from build123d import *
from build123d.topology import SkipClean

# Parameters (mm, degrees)
EXTRUDE_1_DEPTH                            = 3.9
EXTRUDE_3_DEPTH                            = 20
EXTRUDE_5_DEPTH                            = 20
FILLET_1_R                                 = 0.25
FILLET_1_OF_MIRROR_2_R                     = 0.25
SKETCH_7_R                                 = 5.5
CUT_EXTRUDE_3_DEPTH                        = 69.146236458
MIRROR_3_AT_THE_SECOND_PLANE_COPY_1_SKET_R = 5.5
MIRROR_3_AT_THE_SECOND_PLANE_COPY_1_DEPTH  = 69.146236458
ESQUISSE1_W                                = 44.6
ESQUISSE1_H                                = 40
ENL_V_MAT_EXTRU_1_DEPTH                    = 1.54
ENL_V_START                                = -27.2
ENL_V_MAT_EXTRU_2_DEPTH                    = 54.4
ENL_V_MAT_EXTRU_2_2_DEPTH                  = 7.2
ENL_V_START_2                              = 20
ENL_V_MAT_EXTRU_2_3_DEPTH                  = 7.2
ESQUISSE3_W                                = 50
ESQUISSE3_H                                = 1.36
ENL_V_MAT_EXTRU_3_DEPTH                    = 64.372466761
ESQUISSE4_W                                = 27.815449133
ESQUISSE4_H                                = 40
ENL_V_MAT_EXTRU_4_DEPTH                    = 54.066651895
ESQUISSE5_R                                = 1.75
ENL_V_MAT_EXTRU_5_DEPTH                    = 54.198396436


# Read off the part's stored shape, not the designer's step: Enl_v. mat.-Extru.2
with BuildPart() as part:
    # Sketch 1 → Extrude 1 (new body)
    with BuildSketch(Plane(origin=(0, 0, 0), x_dir=(1, 0, 0), z_dir=(0, 1, 0))):
        with BuildLine():
            Line((-40.6, -27.2), (40.6, -27.2))
            ThreePointArc((40.6, -27.2), (43.428427125, -26.028427125), (44.6, -23.2))
            Line((44.6, -23.2), (44.6, 23.2))
            ThreePointArc((44.6, 23.2), (43.428427125, 26.028427125), (40.6, 27.2))
            Line((40.6, 27.2), (-40.6, 27.2))
            ThreePointArc((-40.6, 27.2), (-43.428427125, 26.028427125), (-44.6, 23.2))
            Line((-44.6, 23.2), (-44.6, -23.2))
            ThreePointArc((-44.6, -23.2), (-43.428427125, -26.028427125), (-40.6, -27.2))
        make_face()
    extrude(amount=EXTRUDE_1_DEPTH)



with BuildPart() as body_2:
    # Sketch 3 → Extrude 3 (new, symmetric)
    with BuildSketch(Plane.XY):
        with BuildLine():
            Line((-47.815262386, -6.499919999), (-45.841869662, -6.499919999))
            ThreePointArc((-45.841869662, -6.499919999), (-44.821869662, -1.3), (-43.801869662, -6.499919999))
            Line((-43.801869662, -6.499919999), (-41.828476938, -6.499919999))
            ThreePointArc((-41.828476938, -6.499919999), (-44.821869662, -0.1), (-47.815262386, -6.499919999))
        make_face()
    extrude_3 = extrude(amount=EXTRUDE_3_DEPTH, both=True)


with BuildPart() as part_1:
    with SkipClean():  # the faces are left unmerged after this step: merging them gives an invalid solid
        add(part.part)

        add(body_2.part)  # Extrude 5 merges body 2
        # Sketch 5 → Extrude 5 (add, symmetric)
        with BuildSketch(Plane.XY):
            with BuildLine():
                Line((-36.641600827, 0.870983001), (-34.6, 0))
                ThreePointArc((-34.6, 0), (-38.684888017, -1.351535806), (-41.039960555, -4.952451312))
                Line((-41.039960555, -4.952451312), (-42.295442046, -4.952451312))
                ThreePointArc((-42.295442046, -4.952451312), (-44.821869662, -1.3), (-47.348297278, -4.952451312))
                Line((-47.348297278, -4.952451312), (-48.60377877, -4.952451312))
                ThreePointArc((-48.60377877, -4.952451312), (-44.732839073, 2.293818231), (-36.641600827, 0.870983001))
            make_face()
        extrude_5 = extrude(amount=EXTRUDE_5_DEPTH, both=True)

    # Fillet 1
    fillet_1_edges = [part_1.edges().sort_by_distance(p)[0] for p in [
        (-45.841869662, -6.499919999, 0),
        (-43.801869662, -6.499919999, 0),
    ]]
    fillet(fillet_1_edges, radius=FILLET_1_R)

    # Mirror 1: Extrude 5 across plane
    with SkipClean():  # the faces are left unmerged after this step: merging them gives an invalid solid
        add(extrude_5.mirror(Plane(origin=(0, 0, 0), x_dir=(0, 0, 1), z_dir=(1, 0, 0))))

    # Mirror 2: Extrude 3 across plane
    with SkipClean():  # the faces are left unmerged after this step: merging them gives an invalid solid
        add(extrude_3.mirror(Plane(origin=(0, 0, 0), x_dir=(0, 0, 1), z_dir=(1, 0, 0))))

    # Fillet 1 of Mirror 2
    fillet_1_of_mirror_2_edges = [part_1.edges().sort_by_distance(p)[0] for p in [
        (45.841869662, -6.499919999, 0),
        (43.801869662, -6.499919999, 0),
    ]]
    fillet(fillet_1_of_mirror_2_edges, radius=FILLET_1_OF_MIRROR_2_R)

    # Sketch 7 → Cut-Extrude 3 (cut, through all)
    with SkipClean():  # the faces are left unmerged after this step: merging them gives an invalid solid
        with BuildSketch(Plane.XY.offset(20)):
            with Locations((-45, -4)):
                Circle(SKETCH_7_R)
        cut_extrude_3 = extrude(amount=CUT_EXTRUDE_3_DEPTH, mode=Mode.SUBTRACT)

    # Mirror 3: Cut-Extrude 3 across plane
    with SkipClean():  # the faces are left unmerged after this step: merging them gives an invalid solid
        add(cut_extrude_3.mirror(Plane(origin=(0, 0, 0), x_dir=(0, 0, 1), z_dir=(1, 0, 0))), mode=Mode.SUBTRACT)

    # Mirror 3 at the second plane: Cut-Extrude 3 across plane
    with SkipClean():  # the faces are left unmerged after this step: merging them gives an invalid solid
        add(cut_extrude_3.mirror(Plane.XY), mode=Mode.SUBTRACT)

    # Mirror 3 at the second plane copy 1 sket → Mirror 3 at the second plane copy 1 (cut, through all)
    with SkipClean():  # the faces are left unmerged after this step: merging them gives an invalid solid
        with BuildSketch(Plane(origin=(0, 0, -20), x_dir=(-1, 0, 0), z_dir=(0, 0, -1))):
            with Locations((-45, -4)):
                Circle(MIRROR_3_AT_THE_SECOND_PLANE_COPY_1_SKET_R)
        extrude(amount=MIRROR_3_AT_THE_SECOND_PLANE_COPY_1_DEPTH, mode=Mode.SUBTRACT)

    # Esquisse1 → Enl_v. mat.-Extru.1 (cut)
    with SkipClean():  # the faces are left unmerged after this step: merging them gives an invalid solid
        with BuildSketch(Plane(origin=(0, 3.9, 0), x_dir=(1, 0, 0), z_dir=(0, 1, 0))):
            with Locations((-22.3, 0)):
                Rectangle(ESQUISSE1_W, ESQUISSE1_H)
        extrude(amount=-ENL_V_MAT_EXTRU_1_DEPTH, mode=Mode.SUBTRACT)

    # Enl_v. mat.-Extru.2 outline → Enl_v. mat.-Extru.2 (cut)
    with SkipClean():  # the faces are left unmerged after this step: merging them gives an invalid solid
        with BuildSketch(Plane.XY.offset(ENL_V_START)):
            with BuildLine():
                Line((0, 3.9), (0, 0))
                Line((0, 0), (34.815449133, 0))
                ThreePointArc((34.815449133, 0), (38.762946625, -1.412512906), (41.03576021, -4.935614887))
                ThreePointArc((41.03576021, -4.935614887), (41.343051607, -5.76290242), (41.828476938, -6.499919999))
                Line((41.828476938, -6.499919999), (42.913896916, -6.499919999))
                ThreePointArc((42.913896916, -6.499919999), (43.148596508, -6.33603679), (43.075589522, -6.059248812))
                ThreePointArc((43.075589522, -6.059248812), (44.821869662, -1.3), (46.568149802, -6.059248812))
                ThreePointArc((46.568149802, -6.059248812), (46.495142816, -6.33603679), (46.729842408, -6.499919999))
                Line((46.729842408, -6.499919999), (47.815262386, -6.499919999))
                ThreePointArc((47.815262386, -6.499919999), (48.623960619, -4.868391822), (48.60377877, -3.047548688))
                ThreePointArc((48.60377877, -3.047548688), (47.293490745, 0.166982283), (44.6, 2.356770326))
                Line((44.6, 2.356770326), (44.6, 3.9))
                Line((44.6, 3.9), (0, 3.9))
            make_face()
        extrude(amount=ENL_V_MAT_EXTRU_2_DEPTH, mode=Mode.SUBTRACT)

    # Enl_v. mat.-Extru.2 2 outline → Enl_v. mat.-Extru.2 2 (cut)
    with SkipClean():  # the faces are left unmerged after this step: merging them gives an invalid solid
        with BuildSketch(Plane.XY.offset(ENL_V_START)):
            with BuildLine():
                Line((0, 0), (0, 3.9))
                Line((0, 3.9), (-44.6, 3.9))
                Line((-44.6, 3.9), (-44.60000095, 1.48543533))
                ThreePointArc((-44.60000095, 1.48543533), (-42.784348631, 1.033973481), (-41.225082782, 0))
                Line((-41.225082782, 0), (0, 0))
            make_face()
        extrude(amount=ENL_V_MAT_EXTRU_2_2_DEPTH, mode=Mode.SUBTRACT)

    # Enl_v. mat.-Extru.2 3 outline → Enl_v. mat.-Extru.2 3 (cut)
    with SkipClean():  # the faces are left unmerged after this step: merging them gives an invalid solid
        with BuildSketch(Plane.XY.offset(ENL_V_START_2)):
            with BuildLine():
                Line((0, 0), (0, 3.9))
                Line((0, 3.9), (-44.6, 3.9))
                Line((-44.6, 3.9), (-44.60000095, 1.48543533))
                ThreePointArc((-44.60000095, 1.48543533), (-42.784348631, 1.033973481), (-41.225082782, 0))
                Line((-41.225082782, 0), (0, 0))
            make_face()
        extrude(amount=ENL_V_MAT_EXTRU_2_3_DEPTH, mode=Mode.SUBTRACT)

    # Esquisse3 → Enl_v. mat.-Extru.3 (cut, through all)
    with SkipClean():  # the faces are left unmerged after this step: merging them gives an invalid solid
        with BuildSketch(Plane.XY.offset(20)):
            with Locations((-25, 1.68)):
                Rectangle(ESQUISSE3_W, ESQUISSE3_H)
        extrude(amount=-ENL_V_MAT_EXTRU_3_DEPTH, mode=Mode.SUBTRACT)

    # Esquisse4 → Enl_v. mat.-Extru.4 (cut, through all)
    with SkipClean():  # the faces are left unmerged after this step: merging them gives an invalid solid
        with BuildSketch(Plane.XZ):
            with Locations((-13.907724567, 0)):
                Rectangle(ESQUISSE4_W, ESQUISSE4_H)
        extrude(amount=-ENL_V_MAT_EXTRU_4_DEPTH, mode=Mode.SUBTRACT)

    # Esquisse5 → Enl_v. mat.-Extru.5 (cut, through all)
    with SkipClean():  # the faces are left unmerged after this step: merging them gives an invalid solid
        with BuildSketch(Plane(origin=(0, 1, 0), x_dir=(1, 0, 0), z_dir=(0, 1, 0))):
            with Locations(Location((-36.905449133, 14.9, 0), (0, 0, 270))):
                Circle(ESQUISSE5_R)
            with Locations(Location((-36.905449133, -15.1, 0), (0, 0, 270))):
                Circle(ESQUISSE5_R)
        extrude(amount=-ENL_V_MAT_EXTRU_5_DEPTH, mode=Mode.SUBTRACT)


solid = part_1.part
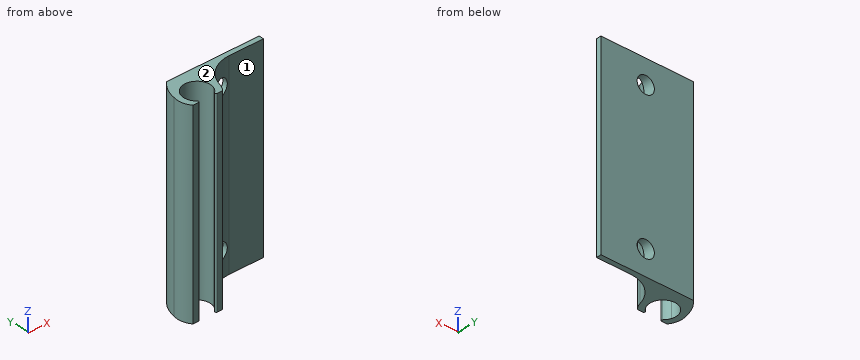
Read the model definition and answer for the solid it produces. Units are mm, in the model's axes. Face numbers are marked on the shaded views. A direction names the side the tool comes from. Coordinates: 2 decimals unless noted, no trailing zeros. Order: outer loops, then holes, each group sorted by start corner. A loop starts at its lowest first (then second) coordinate and runs counter-clockwise, first axis right, second up. Notation, with made-up numbers: M -16.5,68.5 L 13.5,68.5 A24 ccw 13.5,103.5 Z; hole C 29.5,28.25 d2. An arc over 180 degrees is marked long. Put each result on its own line as item: value. Start each with the question number.
Item 1: Given pin 1 Ø6 at (x, z) = (-39, 10) entering from -Y; pin 2 Ø4 at (y, z) = (-5, -6.5) entering from +X; pin 3 Ø3.5 at (x, z) = (-30.5, -3.5) entering from -Y, each flat-ended and moving along its own axis, determine where each tip first touches the part or whether it passes through.
Item 2: Section D-D, the plane z = 18.5 is taken. Determine the outline of the cut face in (x, y).
Item 3: Section C-C, the plane x = -37.5 is taken. Determine the outline of the cut face in (y, z).
Item 4: Section B-B, the plane z = -14.9 is taken. Determine the outline of the cut face in (x, y).
Item 5: For the marked faces 1 and 2, determine the directions among +Z, -Z, +X, -X, +Y, -Y from which every point of the face is accessible in a straight line to the end or side of a thin tool.
Item 6: Section A-A, the plane y = -4.25 is taken. Determine the outline of the cut face in (x, z), plus the area to 3 significant figures.
Item 7: Consider probe 1 along Z at (x, y) = (-38.5, 0.25); probe 2 along X at (y, z) = (-6, 5); probe 3 along Z at (x, y) = (-37.25, -0.25). Determine where each line is inside the solid, lowest interval first. Write a range as [from, to].
Computed:
1. pin 1: stops at y = -6.5
1. pin 2: stops at x = -40.2
1. pin 3: stops at y = 0
2. outline: M -48.6,-3.05 A3.9 ccw -47.82,-6.5 L -46.73,-6.5 A0.25 ccw -46.57,-6.06 A2.7 cw long -43.08,-6.06 A0.25 ccw -42.91,-6.5 L -41.83,-6.5 A3.9 ccw -41.04,-4.94 A6.52 cw -34.82,0 L -27.82,0 L -27.82,1 L -46.57,1 A7 ccw Z
3. outline: M -0.63,-20 L 1,-20 L 1,-16.55 L -0.63,-16.55 Z; M -0.63,-13.25 L 1,-13.25 L 1,13.45 L -0.63,13.45 Z; M -0.63,16.75 L 1,16.75 L 1,20 L -0.63,20 Z
4. outline: M -48.6,-3.05 A3.9 ccw -47.82,-6.5 L -46.73,-6.5 A0.25 ccw -46.57,-6.06 A2.7 cw long -43.08,-6.06 A0.25 ccw -42.91,-6.5 L -41.83,-6.5 A3.9 ccw -41.04,-4.94 A6.52 cw -38.66,-1.33 L -38.66,1 L -46.57,1 A7 ccw Z; M -35.16,-0.01 A6.52 cw -34.82,0 L -27.82,0 L -27.82,1 L -35.16,1 Z
5. face 1: +Z, -Z, +X, -Y
5. face 2: +Z, +X, -X, +Y, -Y
6. outline: M -48.71,-20 L -47.51,-20 L -47.51,20 L -48.71,20 Z; M -42.13,-20 L -40.82,-20 L -40.82,20 L -42.13,20 Z
6. area: 101 mm2
7. probe 1: z = [-20, -15.62], [-14.18, 14.38], [15.82, 20]
7. probe 2: x = [-48.17, -46.64], [-43.01, -41.47]
7. probe 3: z = [-20, -16.62], [-13.18, 13.38], [16.82, 20]
